```python
from build123d import *

# Parameters (mm, degrees)
ESBO_O1_W                = 8.5
ESBO_O1_H                = 8.5
RESSALTO_EXTRUS_O1_DEPTH = 227
FILETE1_R                = 1
FILETE2_R                = 1
FILETE3_R                = 1
ESBO_O2_W                = 215
ESBO_O2_H                = 6.45
CORTE_EXTRUS_O2_DEPTH    = 3.6
ESBO_O3_W                = 3
ESBO_O3_H                = 8.5
RESSALTO_EXTRUS_O3_DEPTH = 10
ESBO_O4_W                = 8.5
ESBO_O4_H                = 3
RESSALTO_EXTRUS_O4_DEPTH = 10
ESBO_O5_W                = 6
ESBO_O5_H                = 2.05
RESSALTO_EXTRUS_O5_DEPTH = 6
ESBO_O6_W                = 2.05
ESBO_O6_H                = 6
RESSALTO_EXTRUS_O6_DEPTH = 6
ESBO_O6_2_W              = 2.05
ESBO_O6_2_H              = 6
RESSALTO_EXTRUS_O7_DEPTH = 6
ESBO_O7_R                = 1.25
CORTE_EXTRUS_O3_DEPTH    = 250
ESBO_O8_R                = 1.25
CORTE_EXTRUS_O4_DEPTH    = 5
ESBO_O9_R                = 1.25
CORTE_EXTRUS_O5_DEPTH    = 5
ESBO_O11_W               = 2.9
ESBO_O11_H               = 13
CORTE_EXTRUS_O6_DEPTH    = 7.7
ESBO_O15_W               = 13
ESBO_O15_H               = 7.7
CORTE_EXTRUS_O10_DEPTH   = 5.9
ESBO_O16_W               = 4
ESBO_O16_H               = 12.5
CORTE_EXTRUS_O12_DEPTH   = 5.9
ESBO_O17_W               = 4
ESBO_O17_H               = 3.401907962
CORTE_EXTRUS_O14_DEPTH   = 0.8


with BuildPart() as part:
    # Esboço1 → Ressalto-extrusão1 (new body)
    with BuildSketch(Plane.XY):
        Rectangle(ESBO_O1_W, ESBO_O1_H)
    extrude(amount=RESSALTO_EXTRUS_O1_DEPTH)

    # Filete1
    filete1_edges = [part.edges().sort_by_distance(p)[0] for p in [
        (4.25, 4.25, 113.5),
    ]]
    fillet(filete1_edges, radius=FILETE1_R)

    # Filete2
    filete2_edges = [part.edges().sort_by_distance(p)[0] for p in [
        (4.25, -0.5, 227),
        (-0.5, 4.25, 227),
        (3.957106781, 3.957106781, 227),
        (-4.25, 0, 227),
        (0, -4.25, 227),
    ]]
    fillet(filete2_edges, radius=FILETE2_R)

    # Filete3
    filete3_edges = [part.edges().sort_by_distance(p)[0] for p in [
        (-0.5, 4.25, 0),
        (3.957106781, 3.957106781, 0),
        (4.25, -0.5, 0),
        (0, -4.25, 0),
        (-4.25, 0, 0),
    ]]
    fillet(filete3_edges, radius=FILETE3_R)

    # Esboço2 → Corte-extrusão2 (cut)
    with BuildSketch(Plane.ZY.offset(4.25)):
        with Locations((113.5, -1.025)):
            Rectangle(ESBO_O2_W, ESBO_O2_H)
    extrude(amount=-CORTE_EXTRUS_O2_DEPTH, mode=Mode.SUBTRACT)

    # Esboço3 → Ressalto-extrusão3 (add)
    with BuildSketch(Plane.ZY.offset(4.25)):
        with Locations((4.5, 0)):
            Rectangle(ESBO_O3_W, ESBO_O3_H)
        with Locations((222.5, 0)):
            Rectangle(ESBO_O3_W, ESBO_O3_H)
    extrude(amount=RESSALTO_EXTRUS_O3_DEPTH)

    # Esboço4 → Ressalto-extrusão4 (add)
    with BuildSketch(Plane.XZ.offset(4.25)):
        with Locations((0, 222.5)):
            Rectangle(ESBO_O4_W, ESBO_O4_H)
        with Locations((0, 4.5)):
            Rectangle(ESBO_O4_W, ESBO_O4_H)
    extrude(amount=RESSALTO_EXTRUS_O4_DEPTH)

    # Esboço5 → Ressalto-extrusão5 (add)
    with BuildSketch(Plane.ZY.offset(4.25)):
        with Locations((9, 3.225)):
            Rectangle(ESBO_O5_W, ESBO_O5_H)
        with Locations((218, 3.225)):
            Rectangle(ESBO_O5_W, ESBO_O5_H)
        with Locations((113.5, 3.225)):
            Rectangle(ESBO_O5_W, ESBO_O5_H)
    extrude(amount=RESSALTO_EXTRUS_O5_DEPTH)

    # Esboço6 → Ressalto-extrusão6 (add)
    with BuildSketch(Plane.XZ.offset(4.25)):
        with Locations((3.225, 9)):
            Rectangle(ESBO_O6_W, ESBO_O6_H)
        Polygon((4.25, 113.5), (4.25, 116.5), (2.2, 116.5), (2.2, 110.5), (4.25, 110.5), align=None)
        with Locations((3.225, 218)):
            Rectangle(ESBO_O6_W, ESBO_O6_H)
    extrude(amount=RESSALTO_EXTRUS_O6_DEPTH)

    # Esboço6<2> → Ressalto-extrusão7 (add)
    with BuildSketch(Plane.XZ.offset(4.25)):
        with Locations((3.225, 9)):
            Rectangle(ESBO_O6_2_W, ESBO_O6_2_H)
        Polygon((4.25, 113.5), (4.25, 116.5), (2.2, 116.5), (2.2, 110.5), (4.25, 110.5), align=None)
        with Locations((3.225, 218)):
            Rectangle(ESBO_O6_2_W, ESBO_O6_2_H)
    extrude(amount=RESSALTO_EXTRUS_O7_DEPTH)

    # Esboço7 → Corte-extrusão3 (cut)
    with BuildSketch(Plane.XY.offset(224)):
        with Locations((-9.25, 0)):
            Circle(ESBO_O7_R)
        with Locations((0, -9.25)):
            Circle(ESBO_O7_R)
    extrude(amount=-CORTE_EXTRUS_O3_DEPTH, mode=Mode.SUBTRACT)

    # Esboço8 → Corte-extrusão4 (cut)
    with BuildSketch(Plane(origin=(4.25, 0, 0), x_dir=(0, 0, -1), z_dir=(1, 0, 0))):
        with Locations((-218.5, -7.25)):
            Circle(ESBO_O8_R)
        with Locations((-113.5, -7.25)):
            Circle(ESBO_O8_R)
        with Locations((-8.5, -7.25)):
            Circle(ESBO_O8_R)
    extrude(amount=-CORTE_EXTRUS_O4_DEPTH, mode=Mode.SUBTRACT)

    # Esboço9 → Corte-extrusão5 (cut)
    with BuildSketch(Plane(origin=(0, 4.25, 0), x_dir=(1, 0, 0), z_dir=(0, 1, 0))):
        with Locations((-7.25, -218.5)):
            Circle(ESBO_O9_R)
        with Locations((-7.25, -113.5)):
            Circle(ESBO_O9_R)
        with Locations((-7.25, -8.5)):
            Circle(ESBO_O9_R)
    extrude(amount=-CORTE_EXTRUS_O5_DEPTH, mode=Mode.SUBTRACT)

    # Esboço11 → Corte-extrusão6 (cut)
    with BuildSketch(Plane.XZ.offset(4.25)):
        with Locations((0.8, 210.578920039)):
            Rectangle(ESBO_O11_W, ESBO_O11_H)
    extrude(amount=-CORTE_EXTRUS_O6_DEPTH, mode=Mode.SUBTRACT)

    # Esboço15 → Corte-extrusão10 (cut)
    with BuildSketch(Plane.ZY.offset(-2.25)):
        with Locations((210.578920039, -0.4)):
            Rectangle(ESBO_O15_W, ESBO_O15_H)
    extrude(amount=CORTE_EXTRUS_O10_DEPTH, mode=Mode.SUBTRACT)

    # Esboço16 → Corte-extrusão12 (cut)
    with BuildSketch(Plane.XZ.offset(-3.45)):
        with Locations((-0.7, 210.328920039)):
            Rectangle(ESBO_O16_W, ESBO_O16_H)
    extrude(amount=-CORTE_EXTRUS_O12_DEPTH, mode=Mode.SUBTRACT)

    # Esboço17 → Corte-extrusão14 (cut)
    with BuildSketch(Plane(origin=(0, 4.25, 0), x_dir=(1, 0, 0), z_dir=(0, 1, 0))):
        with Locations((-0.7, -202.377966058)):
            Rectangle(ESBO_O17_W, ESBO_O17_H)
    extrude(amount=-CORTE_EXTRUS_O14_DEPTH, mode=Mode.SUBTRACT)


solid = part.part
```
Geometry: final body of the model. Coordinates: model frame, mm. A direction names the side the tool comes from. Coordinates: 2 decimals unless noted, no trailing zeros. Order: outer loops, then holes, each group sorted by start corner. A loop starts at its lowest first (then second) coordinate and runs counter-clockwise, first axis right, second up. Notation, with made-up numbers: M 27.5,9 L 45.5,9 A3 cw 45.5,13 Z; hole C 13.25,15 d4. An arc over 180 degrees is marked long. Answer in a Markdown table with one row per item. Add a question column.
Q1. Reachability of faces 1 (the flat face through (2.2, -8, 217)), 2 (the flat face through (-1, 4.25, 112)), 3 (the flat face through (-10.3, -1, 3)), 4 (the flat face through (-1, -10.3, 3)) from +Z, -Z, +X, -X, +Y, -Y: full face, straight path, thin tool, end or side. Return the list, or none.
Q2. Mould query, pull axis Z, two halves, no side actions, for faces 5 (the flat face through (1, 0, 204.079)), 6 (the flat face through (0, 0, 0)), 7 (the flat face through (2, -4.25, 109)), 8 (the flat face through (-10.3, -1, 224)). Classes: released by +Z, released by -Z, zero draft, split by the parting line, or undercut.
Q3. Section query A-A on z = 187. Return the cut outline in (x, y).
Q4. Contact query for flat-ended pins moving along their axis: P1, Ø5, axis at x = -7, y = -12, coming from the -Z side; P2, Ø10, axis at x = -5, z = 39, coming from the -Y side; P3, Ø0.6, axis at y = 3, z = 219, coming from the -X side; P4, Ø0.6, axis at x = -1, y = 4, coming from the -Z side. Output: stop coordinate, or through.
Q5. Line query: L1, parallel to Z at x = -7.25, y = 2.7; L2, parallel to Z at x = -0.25, y = 2.75; L3, parallel to Z at x = -11.5, y = 3.5. Output: solid intervals per line, ascending.
Completed:
| question | item | result |
|---|---|---|
| 1 | face 1 | -X, -Y |
| 1 | face 2 | +Z, -Z, +X, -X, +Y |
| 1 | face 3 | -Z, -X, +Y, -Y |
| 1 | face 4 | -Z, +X, -X, -Y |
| 2 | face 5 | undercut |
| 2 | face 6 | released by -Z |
| 2 | face 7 | undercut |
| 2 | face 8 | released by +Z |
| 3 | outline | M -4.25,2.2 L -0.65,2.2 L -0.65,-4.25 L 4.25,-4.25 L 4.25,3.25 A1 ccw 3.25,4.25 L -4.25,4.25 Z |
| 4 | P1 | passes through |
| 4 | P2 | stops at y = -4.25 |
| 4 | P3 | stops at x = -10.25 |
| 4 | P4 | stops at z = 0.11 |
| 5 | L1 | z = 3 to 7.25, 9.75 to 12, 110.5 to 112.25, 114.75 to 116.5, 215 to 217.25, 219.75 to 224 |
| 5 | L2 | z = 0 to 204.08, 217.08 to 227 |
| 5 | L3 | z = 3 to 6, 221 to 224 |
